```python
from build123d import *

# Parameters (mm, degrees)
SKETCH2_W = 17.145
SKETCH2_H = 11.43


with BuildPart() as part:
    # Sweep1: sweep along a curve in space
    with BuildLine() as sweep1_path:
        Line((0, 0, 0), (59.052587147, 0, 0))
        Line((59.052587147, 0, 0), (59.052587147, 0, -29.66875879))
        Line((59.052587147, 0, -29.66875879), (-4.996664108, 0, -29.66875879))
        Line((-4.996664108, 0, -29.66875879), (-4.996664108, 40.045617421, -29.66875879))
        Line((-4.996664108, 40.045617421, -29.66875879), (-4.996664108, 40.045617421, -60.422953943))
        Line((-4.996664108, 40.045617421, -60.422953943), (-4.996664108, 26.405396034, -60.422953943))
    # Sketch2 → Sweep1 (sweep)
    with BuildSketch(Plane(origin=(0, 0, 0), x_dir=(0, 0, -1), z_dir=(1, 0, 0))):
        Rectangle(SKETCH2_W, SKETCH2_H)
    sweep(path=sweep1_path.line, transition=Transition.RIGHT)


solid = part.part
```
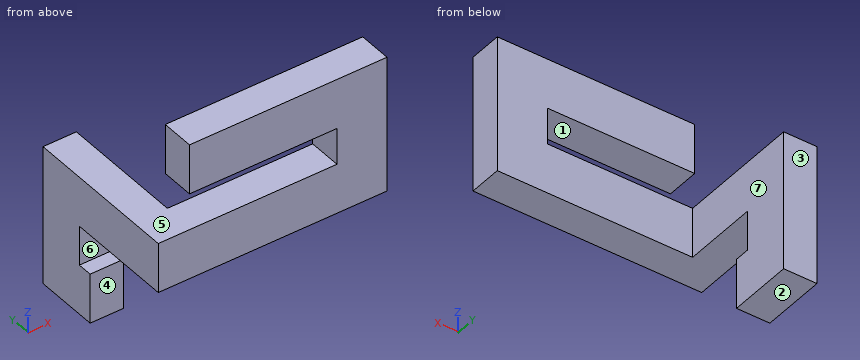
Part model, mm, in its own coordinate system. Face numbers are marked on the shaded views. A direction names the side the tool comes from. Round coordinates to 2 decimals unless told otherwise and drop trailing zeros. Loops run counter-clockwise (first coordinate to the right, second up) from the corner with the lowest first, then second, coordinate; pieces in that order, holes last.
Item 1: 3-axis set-ups, long thin cutter, end or side, ignore diameter. For the marked faces 4, 5, 6 and 7: which of +Z, -Z, +X, -X, +Y, -Y reach the whole face in a straight line?
Item 2: Cut at A-A, the plane x = 18. Give the cut face in (y, z) (1 decimal).
Item 3: Cut at C-C, the plane z = -29.5. Give the cut face in (x, y) (3 decimals), then the cut area to 3 significant figures.
Item 4: Drop flat-ended pins along their axis: P1, Ø3.5, axis at x = -4, z = -59, coming from the -Y side; P2, Ø4, axis at x = -6, y = 29, coming from the +Z side; P3, Ø9, axis at y = -2, z = -12.5, coming from the -X side. Give the stop position or say it passes through.
Item 5: Cut at B-B, the plane y = 28.5. Give the cut face in (x, z), then the cut area to 3 significant figures.
Item 6: Cut at D-D, the plane y = 23. Give the cut face in (x, z), then the cut area to 3 significant figures.
Item 7: Drill centre lines: line 1 (Z direction, x = 6.5, y = 4.5); line 2 (X direction, y = 36.5, z = -52.5); line 3 (Y direction, x = -5.5, z = -49.5). Where is each one in solid material? Low to high.
Item 8: Mould opens along Z. For the marked faces 1, 2 and 3 say: +Z half, -Z half, draft (parallel to the pull), parting line (faces both ways), or undercut.
A:
1. face 4: -Z, +X, -X, -Y
1. face 5: -X, +Y, -Y
1. face 6: +X, -X, -Y
1. face 7: +Z, -Z, +X, +Y
2. outline: (-5.7, -38.2) - (5.7, -38.2) - (5.7, -21.1) - (-5.7, -21.1) - close; (-5.7, -8.6) - (5.7, -8.6) - (5.7, 8.6) - (-5.7, 8.6) - close
3. outline: (-10.712, -5.715) - (67.625, -5.715) - (67.625, 5.715) - (0.718, 5.715) - (0.718, 48.618) - (-10.712, 48.618) - close
3. area: 1,390 mm2
4. P1: stops at y = 26.41
4. P2: stops at z = -21.1
4. P3: stops at x = 0
5. outline: (-10.71, -69) - (0.72, -69) - (0.72, -51.85) - (-10.71, -51.85) - close; (-10.71, -38.24) - (0.72, -38.24) - (0.72, -21.1) - (-10.71, -21.1) - close
5. area: 392 mm2
6. outline: (-10.71, -38.24) - (0.72, -38.24) - (0.72, -21.1) - (-10.71, -21.1) - close
6. area: 196 mm2
7. line 1: z = -38.24 to -21.1, -8.57 to 8.57
7. line 2: x = -10.71 to 0.72
7. line 3: y = 31.47 to 48.62
8. face 1: undercut
8. face 2: -Z half
8. face 3: draft
